For this review, take the finished solid that the model builds, in its own axes (mm). Face numbers are marked on the shaded views. A direction names the side the tool comes from. Give positions to 0.01 mm unless a question says otherwise; leave off trailing zeros. Write each loop counter-clockwise with the first axis right and the second up, starting at its lowest first coordinate (ties: lowest second). Pieces come first, ordered by that corner, then holes. Notation, with made-up numbers: M 47,66.25 L 96,66.25 A20 ccw 96,77.25 Z; hole C 83.25,-20 d5. An arc over 180 degrees is marked long. Answer as a JSON object with one key per item and string values. Group by question number.
```python
from build123d import *

# Parameters (mm, degrees)
F1_DEPTH = 75


with BuildPart() as f1:
    # F0 (on Front) → F1 (new body)
    with BuildSketch(Plane.XZ):
        Polygon((-30, 0), (-25, 0), (-2, 23), (-2, 25), (0, 25), (0, 35), (-2, 35), (-2, 37), (-25, 60), (-30, 60), (-30, 35), (-20, 35), (-20, 25), (-30, 25), align=None)
    extrude(amount=F1_DEPTH)

    # F2: F1 across face


with BuildPart() as f1_1:
    add(f1.part)
    add(f1.part.mirror(Plane(origin=(0, -37.5, 30), x_dir=(0, 1, 0), z_dir=(1, 0, 0))))


solid = f1_1.part
```
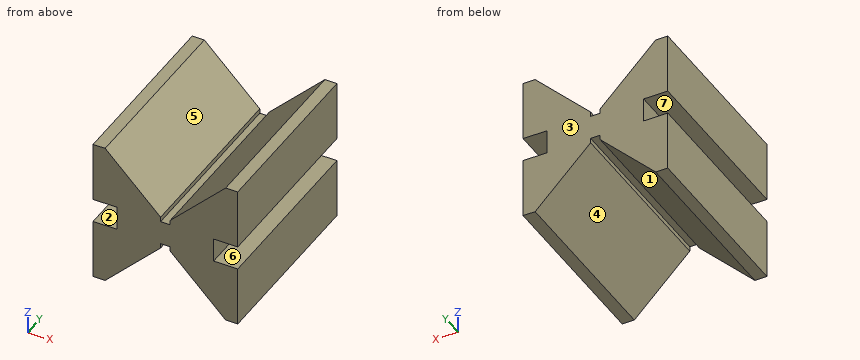
Item 1: Consider section B-B (y = -44.5). Give the boundary of the cut face in (x, z).
Item 2: To check wall thickness, follow probe 1 along X at (y, z) = (-32, 55); probe 2 along X at (y, z) = (-71, 26); probe 3 along X at (y, z) = (-26.5, 42). State the ranges of each line that lie inside material, in increasing order.
Item 3: Consider section D-D (x = 5). Give the boundary of the cut face in (y, z).
Item 4: Draft analysis for pull direction Z (two halves, no side actions). For the marked faces 1, 2 and 3, state which applies: released by +Z, released by -Z, zero draft, split by the parting line, or undercut.
Item 5: Machinability: for the marked faces 4, 5, 6 and 7, which of the approach directions +Z, -Z, +X, -X, +Y, -Y give a long, thin tool a straight path to every point of the face, cutting with its end or side? Answer none if there is none.
Item 6: Consider section C-C (z = 44). Give the boundary of the cut face in (x, y).
Item 7: Insertion check: P1, Ø3, axis at y = -48.5, z = 27.5, coming from the +X side; P2, Ø6, axis at x = 16, y = -14, coming from the +Z side; P3, Ø10, axis at x = 10.5, y = -8, coming from the +Z side. Each pin has a flat end and moves straight along its axis. Give the tip position at first contact, or say it passes through.
Item 8: Consider section A-A (z = 20). Give the boundary of the cut face in (x, y).
Result set:
{
 "1": {"outline": "M -30,0 L -25,0 L -2,23 L -2,25 L 2,25 L 2,23 L 25,0 L 30,0 L 30,25 L 20,25 L 20,35 L 30,35 L 30,60 L 25,60 L 2,37 L 2,35 L -2,35 L -2,37 L -25,60 L -30,60 L -30,35 L -20,35 L -20,25 L -30,25 Z"},
 "2": {"probe 1": "x = -30 to -20, 20 to 30", "probe 2": "x = -20 to 20", "probe 3": "x = -30 to -7, 7 to 30"},
 "3": {"outline": "M -75,20 L 0,20 L 0,40 L -75,40 Z"},
 "4": {"face 1": "released by -Z", "face 2": "undercut", "face 3": "zero draft"},
 "5": {"face 4": "-Z, +Y, -Y", "face 5": "+Z, +Y, -Y", "face 6": "+X, +Y, -Y", "face 7": "-X, +Y, -Y"},
 "6": {"outline": "M -30,-75 L -9,-75 L -9,0 L -30,0 Z; M 9,-75 L 30,-75 L 30,0 L 9,0 Z"},
 "7": {"P1": "stops at x = 20", "P2": "stops at z = 54", "P3": "stops at z = 50.5"},
 "8": {"outline": "M -30,-75 L -5,-75 L -5,0 L -30,0 Z; M 5,-75 L 30,-75 L 30,0 L 5,0 Z"}
}
